from build123d import *

# Parameters (mm, degrees)
F1_DEPTH = 40
F2_R     = 9
F3_DEPTH = 40
F4_R     = 9
F5_DEPTH = 132.5
F7_DEPTH = 100
F6_R     = 10
F9_R     = 10


with BuildPart() as f1:
    # F0 (on Front) → F1 (new body, symmetric)
    with BuildSketch(Plane.XZ):
        Polygon((-10, 10), (0, 0), (58, 0), (58, 40), (18, 40), (18, 80), (-50, 80), (-50, 10), align=None)
    extrude(amount=F1_DEPTH, both=True)

    # F2 (on face) → F3 (join)
    with BuildSketch(Plane.YZ.offset(58)):
        with BuildLine():
            Line((20, 40), (20, 60))
            ThreePointArc((20, 60), (0, 80), (-20, 60))
            Line((-20, 60), (-20, 40))
            Line((-20, 40), (-40, 40))
            Line((-40, 40), (-40, 0))
            Line((-40, 0), (40, 0))
            Line((40, 0), (40, 40))
            Line((40, 40), (20, 40))
        make_face()
        with Locations((0, 60)):
            Circle(F2_R, mode=Mode.SUBTRACT)
    extrude(amount=-F3_DEPTH)


with BuildPart() as f5:
    # F4 (on face) → F5 (new body)
    with BuildSketch(Plane.YZ.offset(18)):
        with Locations((0, 60)):
            Circle(F4_R)
    extrude(amount=-F5_DEPTH)


with BuildPart() as f7:
    # F6 (on face) → F7 (new body)
    with BuildSketch(Plane.XY.offset(80)):
        Polygon((-50, 20), (-50, 0), (-50, -20), (-38, -25), (-38, 25), align=None)
    extrude(amount=-F7_DEPTH)


with BuildPart() as f7b:
    # F6 (on face) → F7, piece 2 (new body)
    with BuildSketch(Plane.XY.offset(80)):
        with Locations((-5, 0)):
            Circle(F6_R)
    extrude(amount=-F7_DEPTH)


with BuildPart() as f1_1:
    add(f1.part)

    # F8: cut F5, F7, F7b
    add(f5.part, mode=Mode.SUBTRACT)
    add(f7.part, mode=Mode.SUBTRACT)
    add(f7b.part, mode=Mode.SUBTRACT)

    # F9
    f9_edges = [f1_1.edges().sort_by_distance(p)[0] for p in [
        (38, -20, 40),
        (38, 20, 40),
    ]]
    fillet(f9_edges, radius=F9_R)


solid = f1_1.part
The listing builds one solid part. Answer for the finished solid, in the listing's coordinates (mm). A direction names the side the tool comes from. Give positions to 0.01 mm unless a question says otherwise; leave off trailing zeros. Order: outer loops, then holes, each group sorted by start corner. A loop starts at its lowest first (then second) coordinate and runs counter-clockwise, first axis right, second up. Notation, with made-up numbers: (-35, -17) - (-9, -17) arc R18 ccw to (-9, -10) - close; hole circle Ø6 at (49.25, 34). An arc over 180 degrees is marked (long way). One line per item, written item: value. Start each with the question number.
1) Find the intervals of material crossed by L1, parallel to Z at x = -25, y = 0; L2, parallel to Z at x = 52.5, y = 0; L3, parallel to Y at x = -28, z = 60, in increasing order.
2) Given pin 1 Ø5 at (x, z) = (29, 53.5) entering from +Y; pin 2 Ø11 at (x, y) = (38, -33.5) entering from +Z; pin 3 Ø16 at (y, z) = (0, 60) entering from -X; pin 4 Ø8 at (x, y) = (-0.5, -11) entering from -Z, each flat-ended and moving along its own axis, determine where each tip first touches the part or whether it passes through.
3) A cutting plane is placed at C-C on x = -5. Give the vertices of the cut face in (y, z), then the cut area to 3 significant figures.
4) A cutting plane is placed at D-D on y = 2. Give the vertices of the cut face in (x, z), then the cut area to 3 significant figures.
5) A tool of negligible diameter and unlimited length cuts with its end or side. For faces 4 (the face through (-38, 0, 45)), 5 (the face through (37.72, 22.85, 43.01)), 6 (the face through (37.72, -22.85, 43.01)), from which of +Z, -Z, +X, -X, +Y, -Y can it reach the whole face along a straight path? Write none if from no direction.
6) A cutting plane is placed at B-B on x = 50. Give the vertices of the cut face in (y, z).
7) The mould has two halves that part along X. Classify faces 1 (the face through (-5, 24, 5)), 2 (the face through (-44.084, -22.465, 45.49)), 3 (the face through (-16, -1, 80)): released by +X, released by -X, zero draft, split by the parting line, or undercut.
8) A cutting plane is placed at A-A on z = 25.5. Give the vertices of the cut face in (x, y).
Answer sheet:
1. L1: z = 10 to 51, 69 to 80
1. L2: z = 0 to 51, 69 to 80
1. L3: y = -40 to -9, 9 to 40
2. pin 1: stops at y = 20
2. pin 2: stops at z = 40.2
2. pin 3: passes through
2. pin 4: stops at z = 0
3. outline: (-40, 5) - (-10, 5) - (-10, 80) - (-40, 80) - close; (10, 5) - (40, 5) - (40, 80) - (10, 80) - close
3. area: 4,500 mm2
4. outline: (-38, 10) - (-14.8, 10) - (-14.8, 51.23) - (-38, 51.23) - close; (-38, 68.77) - (-14.8, 68.77) - (-14.8, 80) - (-38, 80) - close; (4.8, 0) - (58, 0) - (58, 51.23) - (4.8, 51.23) - close; (4.8, 68.77) - (58, 68.77) - (58, 79.9) - (18, 79.9) - (18, 80) - (4.8, 80) - close
4. area: 4,540 mm2
5. face 4: +Z, -Z
5. face 5: +Z, +X, +Y
5. face 6: +Z, +X, -Y
6. outline: (-40, 0) - (40, 0) - (40, 40) - (30, 40) arc R10 cw to (20, 50) - (20, 60) arc R20 ccw to (-20, 60) - (-20, 50) arc R10 cw to (-30, 40) - (-40, 40) - close; hole circle Ø18 at (0, 60)
7. face 1: released by -X
7. face 2: undercut
7. face 3: zero draft
8. outline: (-50, -40) - (58, -40) - (58, 40) - (-50, 40) - (-50, 20) - (-38, 25) - (-38, -25) - (-50, -20) - close; hole circle Ø20 at (-5, 0)
